```python
from build123d import *

# Parameters (mm, degrees)
BOSS_EXTRUDE1_DEPTH      = 20
BOSS_EXTRUDE1_DEPTH_BACK = 15
SKETCH2_R                = 18.2
SKETCH3_R                = 6.5
CUT_EXTRUDE1_DEPTH       = 55


with BuildPart() as part:
    # Sketch1 → Revolve1 (revolve)
    with BuildSketch(Plane.XY):
        Polygon((0, 0), (180, 0), (180, 7.5), (0, 7.5), (0, 10), (-50, 10), (-50, 0), align=None)
    revolve(axis=Axis((0, 0, 0), (-1, 0, 0)))

    # Sketch2 → Boss-Extrude1 (add, two sides: drawn at the far end of the back side and taken through both)
    with BuildSketch(Plane(origin=(0, 0, 0), x_dir=(1, 0, 0), z_dir=(0, 1, 0)).offset(-BOSS_EXTRUDE1_DEPTH_BACK)):
        with Locations(Location((-65, 0, 0), (0, 0, 270))):
            Circle(SKETCH2_R)
    extrude(amount=BOSS_EXTRUDE1_DEPTH + BOSS_EXTRUDE1_DEPTH_BACK)

    # Sketch3 → Cut-Extrude1 (cut)
    with BuildSketch(Plane(origin=(0, 20, 0), x_dir=(1, 0, 0), z_dir=(0, 1, 0))):
        with Locations(Location((-65, 0, 0), (0, 0, 270))):
            Circle(SKETCH3_R)
    extrude(amount=-CUT_EXTRUDE1_DEPTH, mode=Mode.SUBTRACT)


solid = part.part
```
Geometry: final body of the model. Coordinates: model frame, mm. A direction names the side the tool comes from. Give positions to 0.01 mm unless a question says otherwise; leave off trailing zeros. Write each loop counter-clockwise with the first axis right and the second up, starting at its lowest first coordinate (ties: lowest second). Pieces come first, ordered by that corner, then holes.
1. Line query: probe 1 along X at (y, z) = (-0.5, 0); probe 2 along X at (y, z) = (13, 0); probe 3 along Z at (x, y) = (36, -0.5). Output: solid intervals per line, ascending.
2. Draft query along X for faces 3 (the flat face through (-65, 20, 8)), 4 (the cylindrical face through (-71.345, 2.745, -1.409)), 5 (the cylindrical face through (-82.767, 2.255, -3.945)), 6 (the flat face through (180, 0, 0)). Return one class per face: released by +X, released by -X, zero draft, split by the parting line, or undercut.
3. Section query B-B, the plane y = 0. Return loops of the section in (x, z).
4. Section query D-D, the plane x = 112.5. Return loops of the section in (y, z).
5. Section query A-A, the plane z = 0. Return loops of the section in (x, y), then the cut area to 4 significant figures.
6. Section query C-C, the plane x = -65. Return loops of the section in (y, z), then the cut area to 3 significant figures.
7. Reachability of faces 1 (the flat face through (0, -4, -7)), 2 (the flat face through (-65, -15, 8)) from +Z, -Z, +X, -X, +Y, -Y: full face, straight path, thin tool, end or side. Return the list, or none.
8. Pin query (flat end, axial travel): P1, Ø2, axis at x = 8.5, z = 3, coming from the -Y side; P2, Ø1, axis at x = -24.5, z = -3, coming from the -Y side; P3, Ø5, axis at x = 39.5, y = -9, coming from the -Z side. Return the tip coordinate at first contact, or that it passes through.
Computed:
1. probe 1: x = -83.2 to -71.5, -58.5 to 180
1. probe 2: x = -83.2 to -71.5, -58.5 to -46.8
1. probe 3: z = -7.48 to 7.48
2. face 3: zero draft
2. face 4: undercut
2. face 5: split by the parting line
2. face 6: released by +X
3. outline: (-49.79, -10) - (0, -10) - (0, -7.5) - (180, -7.5) - (180, 7.5) - (0, 7.5) - (0, 10) - (-49.79, 10) arc R18.2 ccw (long way) to start; hole circle Ø13 at (-65, 0)
4. outline: circle Ø15 at (0, 0)
5. outline: (-83.2, -15) - (-71.5, -15) - (-71.5, 20) - (-83.2, 20) - close; (-58.5, -15) - (-46.8, -15) - (-46.8, -10) - (0, -10) - (0, -7.5) - (180, -7.5) - (180, 7.5) - (0, 7.5) - (0, 10) - (-46.8, 10) - (-46.8, 20) - (-58.5, 20) - close
5. area: 4,455 mm2
6. outline: (-15, -18.2) - (20, -18.2) - (20, -6.5) - (-15, -6.5) - close; (-15, 6.5) - (20, 6.5) - (20, 18.2) - (-15, 18.2) - close
6. area: 819 mm2
7. face 1: +X
7. face 2: +Z, -Z, +X, -X, -Y
8. P1: stops at y = -7.23
8. P2: stops at y = -9.68
8. P3: stops at z = -3.74
